Build history of the part. All positions in model axes, mm. A direction names the side the tool comes from. Round coordinates to 2 decimals unless told otherwise and drop trailing zeros. Write each loop counter-clockwise with the first axis right and the second up, starting at its lowest first coordinate (ties: lowest second). Pieces come first, ordered by that corner, then holes.
1) Which spindle directions (+Z, -Z, +X, -X, +Y, -Y) get a long thin tool onto all of the face, cutting with end or side? Do faces 1 (the flat face through (0.45, 2, 1)), 2 (the cylindrical face through (0.45, -2.96, -1.43)), 3 (the flat face through (0, -6, 0)). Say none if no direction does.
2) Flat gauge pins, fed straight in: pin 1 (1.6 mm diameter, centred on x = -1, y = 2.5, fed in from +Z); pin 2 (1.2 mm diameter, centred on y = 2, z = -1.5, fed in from -X); pin 3 (1.2 mm diameter, centred on y = 2.5, z = 1.5, fed in from +X). Where does each tip first touch, or does it go through?
3) Pull direction Z, two halves, no side cores. Call faces 4 (the cylindrical face through (0.9, 0.89, 2.86)), 5 (the flat face through (-1, 2, -0.45)), 6 (the flat face through (1, 3, -1)): +Z half, -Z half, draft (parallel to the pull), parting line (faces both ways), or undercut.
4) Wall check: probe 1 along Y at (x, z) = (0.25, 1.75); probe 2 along Y at (x, z) = (0.5, -0.25); probe 3 along Z at (x, y) = (0.5, 1.75). Give the ranges that are in metal, low to high.
5) Saw through at A-A (y = -2). Write the cut outline in (x, z), plus the area to 3 significant figures.
from build123d import *

# Parameters (mm, degrees)
SKETCH1_R           = 3
BOSS_EXTRUDE1_DEPTH = 3
SKETCH2_R           = 1.5
BOSS_EXTRUDE2_DEPTH = 6
CUT_EXTRUDE1_DEPTH  = 1.5
FILLET1_SIZE        = 1.2
FILLET1_SIZE_2      = 0.6


with BuildPart() as part:
    # Sketch1 → Boss-Extrude1 (new body)
    with BuildSketch(Plane(origin=(0, 0, 0), x_dir=(1, 0, 0), z_dir=(0, 1, 0))):
        with Locations(Location((0, 0, 0), (0, 0, 270))):
            Circle(SKETCH1_R)
    extrude(amount=BOSS_EXTRUDE1_DEPTH)

    # Sketch2 → Boss-Extrude2 (add)
    with BuildSketch(Plane.XZ):
        with Locations(Location((0, 0, 0), (0, 0, 270))):
            Circle(SKETCH2_R)
    extrude(amount=BOSS_EXTRUDE2_DEPTH)

    # Sketch3 → Cut-Extrude1 (cut)
    with BuildSketch(Plane(origin=(0, 3, 0), x_dir=(1, 0, 0), z_dir=(0, 1, 0))):
        Polygon((-0.45, 2.25), (-0.45, 0.45), (-2.25, 0.45), (-2.25, -0.45), (-0.45, -0.45), (-0.45, -2.25), (0.45, -2.25), (0.45, -0.45), (2.25, -0.45), (2.25, 0.45), (0.45, 0.45), (0.45, 2.25), align=None)
    extrude(amount=-CUT_EXTRUDE1_DEPTH, mode=Mode.SUBTRACT)

    # Fillet1
    # an asymmetric fillet: 1.2, 0.6 mm, written as the material it takes off along each edge
    with BuildSketch(Plane(origin=(0, 3, 0), x_dir=(0, 0, 1), z_dir=(-1, 0, 0))) as fillet1_piece_1:
        with BuildLine():
            Bezier((3, -FILLET1_SIZE), (3, 0), (3 - FILLET1_SIZE_2, 0), weights=[1, 0.707106781, 1])
            Line((3 - FILLET1_SIZE_2, 0), (3, 0))
            Line((3, 0), (3, -FILLET1_SIZE))
        make_face()
    revolve(axis=Axis((0, 3, 0), (0, 1, 0)), mode=Mode.SUBTRACT)


solid = part.part
Evaluation:
1. face 1: +Y
1. face 2: -Y
1. face 3: +Z, -Z, +X, -X, -Y
2. pin 1: stops at z = 2.97
2. pin 2: stops at x = -2.86
2. pin 3: stops at x = 2.8
3. face 4: parting line
3. face 5: undercut
3. face 6: draft
4. probe 1: y = 0 to 1.5
4. probe 2: y = -6 to 1.5
4. probe 3: z = -2.96 to -0.45, 0.45 to 2.96
5. outline: circle Ø3 at (0, 0)
5. area: 7.07 mm2
